Job drawing, mm, ordinate dimensions from the low corner. One solid piece. A direction names the side the tool comes from. Round coordinates to 2 decimals unless told otherwise and drop trailing zeros. Loops run counter-clockwise (first coordinate to the right, second up) from the corner with the lowest first, then second, coordinate; pieces in that order, holes last. Notation, with made-up numbers: M -18.75,-39 L -10.75,-39 A19 cw -10.75,-35 Z; hole C -17.75,-16 d11. An arc over 180 degrees is marked long. One line per item, written item: value.
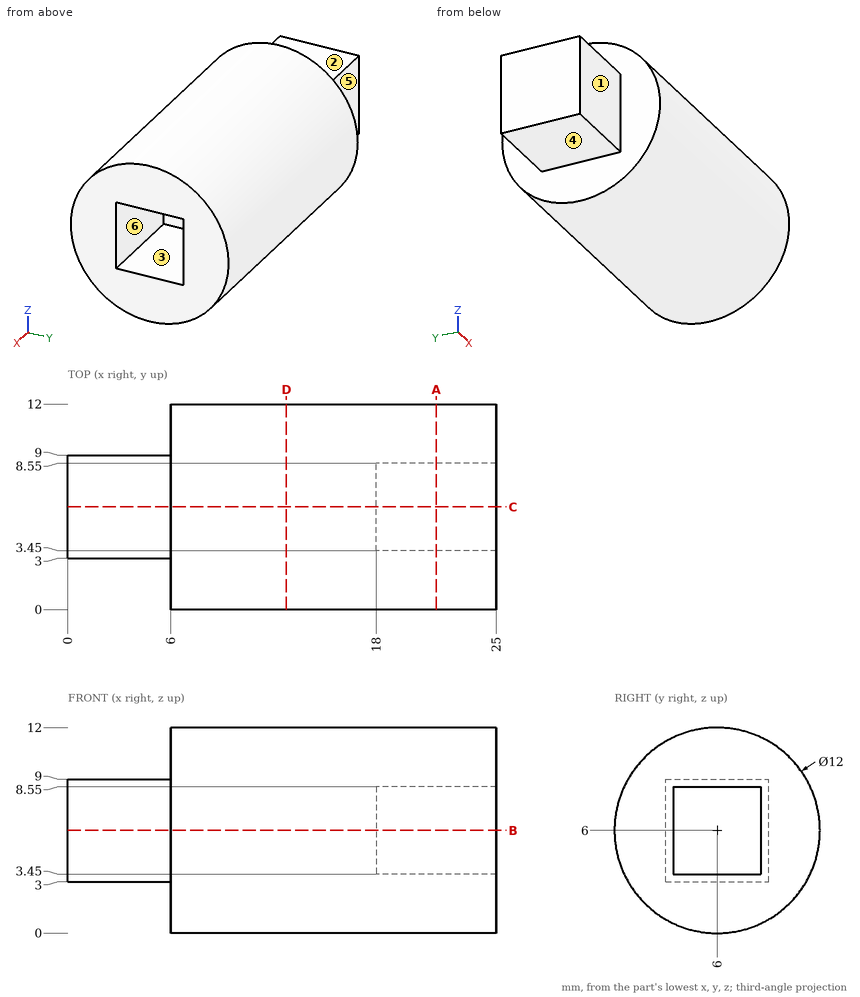
Item 1: Slice it at B-B, the plane z = 6. Give the cut face in (x, y).
Check values:
outline: M 0,3 L 6,3 L 6,0 L 25,0 L 25,3.45 L 18,3.45 L 18,8.55 L 25,8.55 L 25,12 L 6,12 L 6,9 L 0,9 Z
Item 2: Slice it at D-D, the plane x = 12.75. Give the cut face in (y, z).
Check values:
outline: C 6,6 d12
Item 3: Drop flat-ended pins along their axis: P1, Ø1, axis at y = 4.5, z = 3.5, coming from the +X side; P2, Ø3, axis at x = 4, z = 5, coming from the -Y side; P3, Ø3, axis at x = 5, y = 10.5, coming from the -Z side; P4, Ø1, axis at x = 10.5, y = 5, coming from the +Z side. Give the stop position or say it passes through.
Check values:
P1: stops at x = 25
P2: stops at y = 3
P3: stops at z = 1.04
P4: stops at z = 11.98
Item 4: Which spindle directions (+Z, -Z, +X, -X, +Y, -Y) get a long thin tool onto all of the face, cutting with end or side? Do the marked faces 1, 2 and 3. Say none if no direction does.
Check values:
face 1: +Z, -Z, -X, -Y
face 2: +Z, -X, +Y, -Y
face 3: +X
Item 5: Slice it at A-A, the plane x = 21.5. Give the cut face in (y, z).
Check values:
outline: C 6,6 d12; hole M 3.45,3.45 L 8.55,3.45 L 8.55,8.55 L 3.45,8.55 Z
Item 6: Wall check: line 1 along X through (y, z) = (8.5, 10.5); line 2 along Y through (x, z) = (5.5, 5.5); line 3 along Z through (x, y) = (20.75, 7.75). Give the ranges that are in metal, low to high.
Check values:
line 1: x = 6 to 25
line 2: y = 3 to 9
line 3: z = 0.26 to 3.45, 8.55 to 11.74
Item 7: Pull direction Z, two halves, no side cores. Call the marked faces 4, 5 and 6: pulls with the +Z half, pulls with the -Z half, needs draft (parallel to the pull), parting line crosses it, or undercut.
Check values:
face 4: pulls with the -Z half
face 5: needs draft
face 6: undercut
